Build history of the part. All positions in model axes, mm. A direction names the side the tool comes from. Coordinates: 2 decimals unless noted, no trailing zeros. Order: outer loops, then holes, each group sorted by start corner. A loop starts at its lowest first (then second) coordinate and runs counter-clockwise, first axis right, second up. Notation, with made-up numbers: (89.5, -13.5) - (139.5, -13.5) arc R13 cw to (139.5, -7.5) - close; hole circle Ø6 at (-5, 52.5). An arc over 180 degrees is marked (long way). One line per item, written item: value.
from build123d import *

# Parameters (mm, degrees)
SKETCH1_W           = 88.9
SKETCH1_H           = 31.75
BOSS_EXTRUDE1_DEPTH = 7.62
CUT_EXTRUDE1_DEPTH  = 29.464
CUT_EXTRUDE2_DEPTH  = 29.464
SKETCH4_R           = 1.27
CUT_EXTRUDE3_DEPTH  = 7.62
SKETCH5_R           = 1.27
CUT_EXTRUDE4_DEPTH  = 7.62


with BuildPart() as part:
    # Sketch1 → Boss-Extrude1 (new body)
    with BuildSketch(Plane(origin=(0, 0, 0), x_dir=(1, 0, 0), z_dir=(0, 1, 0))):
        Rectangle(SKETCH1_W, SKETCH1_H)
    extrude(amount=BOSS_EXTRUDE1_DEPTH)

    # Sketch2 → Cut-Extrude1 (cut)
    with BuildSketch(Plane(origin=(0, 7.62, 0), x_dir=(1, 0, 0), z_dir=(0, 1, 0))):
        Polygon((-38.1, 3.175), (-38.1, 13.335), (-2.563992866, 13.335), align=None)
        Polygon((-38.1, -3.175), (-38.1, -13.335), (-2.563992866, -13.335), align=None)
        Polygon((2.54, 13.335), (38.1, 13.335), (38.1, 3.175), align=None)
        Polygon((38.1, -3.175), (38.1, -13.335), (2.54, -13.335), align=None)
    extrude(amount=-CUT_EXTRUDE1_DEPTH, mode=Mode.SUBTRACT)

    # Sketch3 → Cut-Extrude2 (cut)
    with BuildSketch(Plane(origin=(0, 7.62, 0), x_dir=(1, 0, 0), z_dir=(0, 1, 0))):
        Polygon((0, 9.525), (-24.292421741, 0), (0, -9.525), (26.507578259, 0), align=None)
    extrude(amount=-CUT_EXTRUDE2_DEPTH, mode=Mode.SUBTRACT)

    # Sketch4 → Cut-Extrude3 (cut)
    with BuildSketch(Plane(origin=(44.45, 0, 0), x_dir=(0, 0, -1), z_dir=(1, 0, 0))):
        with Locations((0, 3.786925891)):
            Circle(SKETCH4_R)
    extrude(amount=-CUT_EXTRUDE3_DEPTH, mode=Mode.SUBTRACT)

    # Sketch5 → Cut-Extrude4 (cut)
    with BuildSketch(Plane.ZY.offset(44.45)):
        with Locations((0, 3.81)):
            Circle(SKETCH5_R)
    extrude(amount=-CUT_EXTRUDE4_DEPTH, mode=Mode.SUBTRACT)


solid = part.part
1. Band-saw the part on A-A, the plane x = 32. Give the cut face in (y, z) (3 decimals), and give its area (3 significant figures).
Values found:
outline: (0, -15.875) - (7.62, -15.875) - (7.62, -13.335) - (0, -13.335) - close; (0, -4.918) - (7.62, -4.918) - (7.62, 4.918) - (0, 4.918) - close; (0, 13.335) - (7.62, 13.335) - (7.62, 15.875) - (0, 15.875) - close
area: 114 mm2
2. 3-axis set-ups, long thin cutter, end or side, ignore diameter. For faces 4 (the face through (20.071, 3.863, 8.326)), 5 (the face through (36.83, 4, 0)), 6 (the face through (-36.83, 4, 0)): which of +Z, -Z, +X, -X, +Y, -Y reach the whole face in a straight line?
Values found:
face 4: +Y, -Y
face 5: +X
face 6: -X
3. Band-saw the part on B-B, the plane z = -11.5. Give the cut face in (x, y), and give its area (3 significant figures).
Values found:
outline: (-44.45, 0) - (-38.1, 0) - (-38.1, 7.62) - (-44.45, 7.62) - close; (-8.98, 0) - (8.96, 0) - (8.96, 7.62) - (-8.98, 7.62) - close; (38.1, 0) - (44.45, 0) - (44.45, 7.62) - (38.1, 7.62) - close
area: 234 mm2
4. Flat gauge pin, fed straight in: P1, Ø0.8, axis at y = 3.5, z = 0, coming from the -X side. Where does the tip first touch, or does it go through?
Values found:
P1: stops at x = -36.83
5. Probe line 1 along Y through (x, z) = (40, 0); line 2 along Z through (x, y) = (-26, 5.25) (3 decimals); line 3 along Z through (x, y) = (17, 2.75) (3 decimals). List the from-to ranges inside material, lowest first.
Values found:
line 1: y = 0 to 2.52, 5.06 to 7.62
line 2: z = -15.875 to -13.335, -6.634 to 6.634, 13.335 to 15.875
line 3: z = -15.875 to -13.335, -9.204 to -3.416, 3.416 to 9.204, 13.335 to 15.875
6. Band-saw the part on D-D, the plane x = 4.5. Give the cut face in (y, z) (3 decimals).
Values found:
outline: (0, -15.875) - (7.62, -15.875) - (7.62, -13.335) - (0, -13.335) - close; (0, -12.775) - (7.62, -12.775) - (7.62, -7.908) - (0, -7.908) - close; (0, 7.908) - (7.62, 7.908) - (7.62, 12.775) - (0, 12.775) - close; (0, 13.335) - (7.62, 13.335) - (7.62, 15.875) - (0, 15.875) - close
7. Band-saw the part on C-C, the plane y = 1.5. Give the cut face in (x, z) (3 decimals), and give its area (3 significant figures).
Values found:
outline: (-44.45, -15.875) - (44.45, -15.875) - (44.45, 15.875) - (-44.45, 15.875) - close; hole (-38.1, -13.335) - (-2.564, -13.335) - (-38.1, -3.175) - close; hole (-38.1, 3.175) - (-2.564, 13.335) - (-38.1, 13.335) - close; hole (-24.292, 0) - (0, -9.525) - (26.508, 0) - (0, 9.525) - close; hole (2.54, -13.335) - (38.1, -13.335) - (38.1, -3.175) - close; hole (2.54, 13.335) - (38.1, 3.175) - (38.1, 13.335) - close
area: 1,620 mm2
8. Two-plate mould, pull along X, no slides. Class faces 1 (the face through (44.45, 5.4, 0.2)), 2 (the face through (-12.316, 3.863, 4.696)), 3 (the face through (40.69, 2.55, 0.28)): pulls with the +X half, pulls with the -X half, needs draft (parallel to the pull), parting line crosses it, or undercut.
Values found:
face 1: pulls with the +X half
face 2: undercut
face 3: needs draft
